Geometry: see drawing. Coordinates: mm, zero at the bounding-box minimum. Give positions to 0.01 mm unless a question says otherwise; leave off trailing zeros. Loops run counter-clockwise (first coordinate to the right, second up) from the corner with the lowest first, then second, coordinate; pieces in that order, holes last. Notation, with made-up numbers: (-3.5, -25) - (14.5, -25) arc R20 cw to (14.5, -15) - close; hole circle Ø9 at (-10, 49). An arc over 180 degrees is marked (long way). One line per question, with ' | ' between items. Start each with the question number.
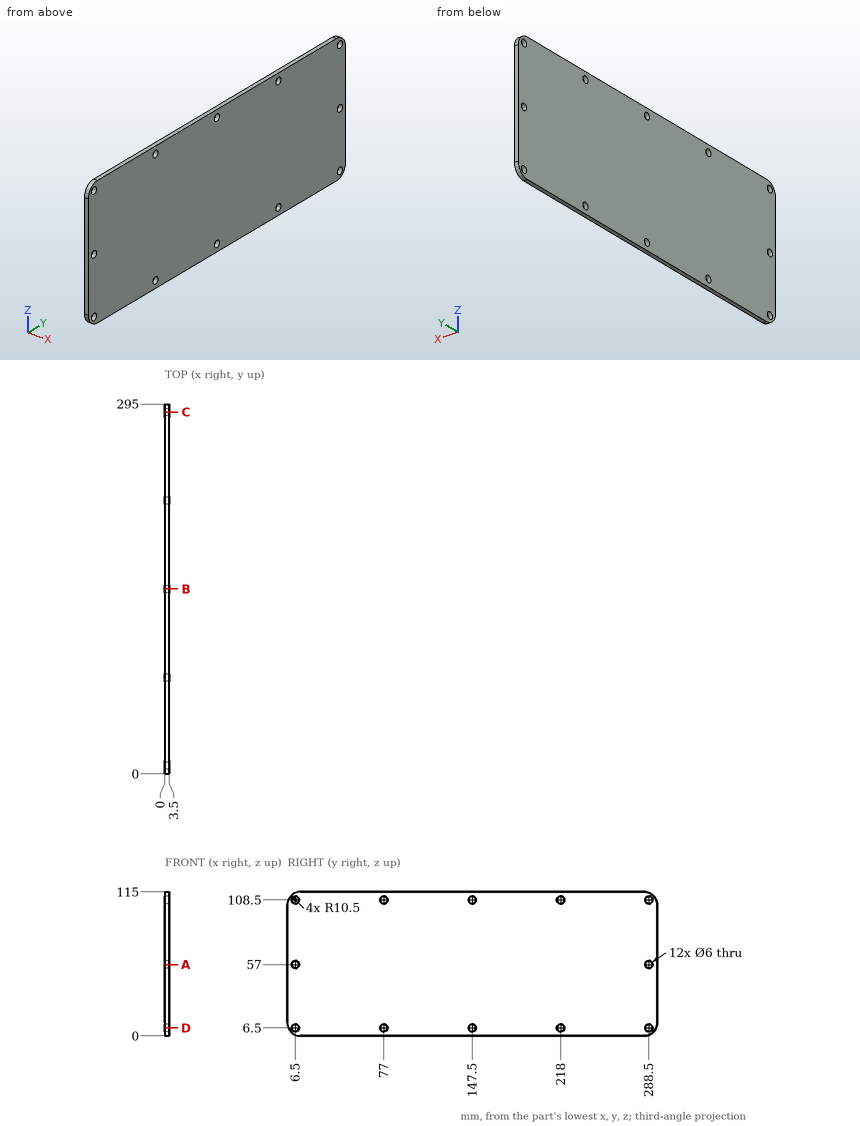
Q1. First-contact query: pin 1 (3.5 mm diameter, centred on y = 288.5, z = 108.5, fed in from -X). Flat tip, straight axial feed; report the tip coordinate or a pass-through.
Q2. Section D-D, the plane z = 6.5. Output: boundary loops of the cut face in (x, y).
Q3. Section B-B, the plane y = 147.5. Output: boundary loops of the cut face in (x, z).
Q4. Section A-A, the plane z = 57. Output: boundary loops of the cut face in (x, y), plus the area to 4 significant figures.
Q5. Section C-C, the plane y = 288.5. Output: boundary loops of the cut face in (x, z), plus the area to 3 significant figures.
Q6. Line query: L1, parallel to Z at x = 0.75, y = 147.5; L2, parallel to Y at x = 1.35, z = 57; L3, parallel to Y at x = 2.45, z = 6.5. Output: solid intervals per line, ascending. Write a range as from..to.
Solved:
1) pin 1: passes through
2) outline: (0, 0.79) - (3.5, 0.79) - (3.5, 3.5) - (0, 3.5) - close; (0, 9.5) - (3.5, 9.5) - (3.5, 74) - (0, 74) - close; (0, 80) - (3.5, 80) - (3.5, 144.5) - (0, 144.5) - close; (0, 150.5) - (3.5, 150.5) - (3.5, 215) - (0, 215) - close; (0, 221) - (3.5, 221) - (3.5, 285.5) - (0, 285.5) - close; (0, 291.5) - (3.5, 291.5) - (3.5, 294.21) - (0, 294.21) - close
3) outline: (0, 0) - (3.5, 0) - (3.5, 3.5) - (0, 3.5) - close; (0, 9.5) - (3.5, 9.5) - (3.5, 105.5) - (0, 105.5) - close; (0, 111.5) - (3.5, 111.5) - (3.5, 115) - (0, 115) - close
4) outline: (0, 0) - (3.5, 0) - (3.5, 3.5) - (0, 3.5) - close; (0, 9.5) - (3.5, 9.5) - (3.5, 285.5) - (0, 285.5) - close; (0, 291.5) - (3.5, 291.5) - (3.5, 295) - (0, 295) - close | area: 990.5 mm²
5) outline: (0, 0.79) - (3.5, 0.79) - (3.5, 3.5) - (0, 3.5) - close; (0, 9.5) - (3.5, 9.5) - (3.5, 54) - (0, 54) - close; (0, 60) - (3.5, 60) - (3.5, 105.5) - (0, 105.5) - close; (0, 111.5) - (3.5, 111.5) - (3.5, 114.21) - (0, 114.21) - close | area: 334 mm²
6) L1: z = 0..3.5, 9.5..105.5, 111.5..115 | L2: y = 0..3.5, 9.5..285.5, 291.5..295 | L3: y = 0.79..3.5, 9.5..74, 80..144.5, 150.5..215, 221..285.5, 291.5..294.21
